Here's how the part is built. I have some questions about the finished solid (model axes, mm). Face numbers are marked on the shaded views. A direction names the side the tool comes from. Give positions to 0.01 mm unless a question says otherwise; leave off trailing zeros. Write each loop counter-clockwise with the first axis right and the second up, starting at its lowest first coordinate (ties: lowest second). Pieces come first, ordered by that corner, then holes. Notation, with made-up numbers: (-29, -26.75) -> (25, -26.75) arc R34 ccw to (25, 3.25) -> close; hole circle Ø11 at (-27.5, 88.25). An arc over 180 degrees is marked (long way). Use one line per item in the form item = value.
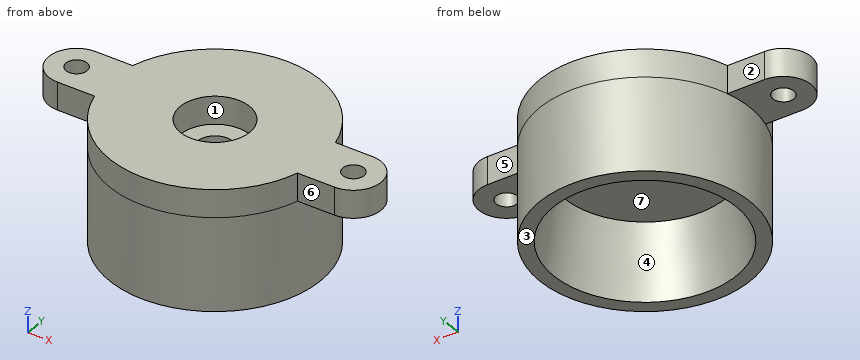
```python
from build123d import *

# Parameters (mm, degrees)
F0_R     = 24.13
F0_R_2   = 20.955
F1_DEPTH = 16.51
F2_R     = 18.415
F2_R_2   = 24.13
F4_DEPTH = 4.7625
F5_R     = 3.96875
F6_DEPTH = 4.7625
F5_R_2   = 2.413
F5_R_3   = 7.9375
F7_DEPTH = 6.35


# Not quite as in the source:
# - a feature names something its author has since deleted; it is built from what else it names


with BuildPart() as f1:
    # F0 (on Top) → F1 (new body)
    with BuildSketch(Plane.XY):
        Circle(F0_R)
        Circle(F0_R_2, mode=Mode.SUBTRACT)
        Circle(F0_R_2)
    extrude(amount=F1_DEPTH)

    # F0 (on Top) → F3 section 0
    with BuildSketch(Plane.XY):
        Circle(F0_R_2)
    # F2 (on face) → F3 section 1
    with BuildSketch(Plane.XY.offset(16.51)):
        Circle(F2_R)
    loft(mode=Mode.SUBTRACT)

    # F2 (on face) → F4 (join)
    with BuildSketch(Plane.XY.offset(16.51)):
        Circle(F2_R_2)
        Circle(F2_R, mode=Mode.SUBTRACT)
        Circle(F2_R)
    extrude(amount=F4_DEPTH)

    # F5 (on face) → F6 (cut, through all)
    with BuildSketch(Plane.XY.offset(21.2725)):
        Circle(F5_R)
    extrude(amount=-F6_DEPTH, mode=Mode.SUBTRACT)

    # F5 (on face) → F7 (join)
    with BuildSketch(Plane.XY.offset(21.2725)):
        with BuildLine():
            Line((-26.2298047315, 6.35), (-31.75, 6.35))
            ThreePointArc((-31.75, 6.35), (-38.1, 0), (-31.75, -6.35))
            Line((-31.75, -6.35), (-26.2298047315, -6.35))
            ThreePointArc((-26.2298047315, -6.35), (-26.9875, 0), (-26.2298047315, 6.35))
        make_face()
        with Locations((-31.75, 0)):
            Circle(F5_R_2, mode=Mode.SUBTRACT)
        with BuildLine():
            ThreePointArc((23.2794845304, 6.35), (0, 24.13), (-23.2794845304, 6.35))
            ThreePointArc((-23.2794845304, 6.35), (-24.13, 0), (-23.2794845304, -6.35))
            ThreePointArc((-23.2794845304, -6.35), (0, -24.13), (23.2794845304, -6.35))
            ThreePointArc((23.2794845304, -6.35), (23.9164259633, -3.2033527968), (24.13, 0))
            ThreePointArc((24.13, 0), (23.9164259633, 3.2033527968), (23.2794845304, 6.35))
        make_face()
        Circle(F5_R_3, mode=Mode.SUBTRACT)
        with BuildLine():
            Line((31.75, 6.35), (26.2298047315, 6.35))
            ThreePointArc((26.2298047315, 6.35), (26.9875, 0), (26.2298047315, -6.35))
            Line((26.2298047315, -6.35), (31.75, -6.35))
            ThreePointArc((31.75, -6.35), (38.1, 0), (31.75, 6.35))
        make_face()
        with Locations((31.75, 0)):
            Circle(F5_R_2, mode=Mode.SUBTRACT)
        with BuildLine():
            Line((-23.2794845304, 6.35), (-26.2298047315, 6.35))
            ThreePointArc((-26.2298047315, 6.35), (-26.9875, 0), (-26.2298047315, -6.35))
            Line((-26.2298047315, -6.35), (-23.2794845304, -6.35))
            ThreePointArc((-23.2794845304, -6.35), (-24.13, 0), (-23.2794845304, 6.35))
        make_face()
        with BuildLine():
            Line((26.2298047315, 6.35), (23.2794845304, 6.35))
            ThreePointArc((23.2794845304, 6.35), (23.9164259633, 3.2033527968), (24.13, 0))
            ThreePointArc((24.13, 0), (23.9164259633, -3.2033527968), (23.2794845304, -6.35))
            Line((23.2794845304, -6.35), (26.2298047315, -6.35))
            ThreePointArc((26.2298047315, -6.35), (26.9875, 0), (26.2298047315, 6.35))
        make_face()
    extrude(amount=F7_DEPTH)


solid = f1.part
```
Q1. I want a section at C-C, the plane z = 18. Write out the boundary of the cut face in (x, y), and give its area (3 significant figures).
Result set:
outline = circle Ø48.26 at (0, 0); hole circle Ø7.94 at (0, 0)
area = 1,780 mm2
Q2. I want a section at D-D, the plane z = 11. Write out the boundary of the cut face in (x, y), and give its area (3 significant figures).
Result set:
outline = circle Ø48.26 at (0, 0); hole circle Ø38.53 at (0, 0)
area = 664 mm2
Q3. Will these pins go through, and if not, where does the flat tip stop? pin 1 Ø8 at (x, z) = (-3, 20.5) entering from -Y; pin 2 Ø5.5 at (x, y) = (31.75, 0) entering from -Z; pin 3 Ø12 at (x, z) = (21, 22.5) entering from +Y.
Result set:
pin_1 = -24.13
pin_2 = 21.27
pin_3 = 18.9
Q4. I want a section at A-A, the plane x = 0. Write out the boundary of the cut face in (y, z) (1 decimal), and give its area (3 significant figures).
Result set:
outline = (-24.1, 0) -> (-21, 0) -> (-18.4, 16.5) -> (-4, 16.5) -> (-4, 21.3) -> (-7.9, 21.3) -> (-7.9, 27.6) -> (-24.1, 27.6) -> close; (4, 16.5) -> (18.4, 16.5) -> (21, 0) -> (24.1, 0) -> (24.1, 27.6) -> (7.9, 27.6) -> (7.9, 21.3) -> (4, 21.3) -> close
area = 544 mm2
Q5. If I drill on line 1 along Y through (x, z) = (0, 19.5); line 2 along Y through (x, z) = (0, 24.5); line 3 along X through (y, z) = (-2.5, 5.5), over which ranges is the centre line in solid material (lowest first)? Write a range as from..to.
Result set:
line_1 = -24.13..-3.97, 3.97..24.13
line_2 = -24.13..-7.94, 7.94..24.13
line_3 = -24..-19.95, 19.95..24
Q6. Which directions (+Z, -Z, +X, -X, +Y, -Y) give clear straight access to the entire face, cutting with the end or side of a thin tool? Please do the marked faces 5, 6 and 7.
Result set:
face_5 = +Z, -Z, +X, +Y
face_6 = +Z, -Z, +X, -Y
face_7 = -Z
Q7. I want a section at B-B, the plane y = 0. Count the separate pieces of the cut face and the enclosed holes in it, and give its area (3 significant figures).
Result set:
separate_pieces = 4
enclosed_holes = 0
area = 661 mm2
Q8. If we mould it in two halves opening along Y, with no side actions, what happens to the marked faces 1, 2, 3 and 4? For each: +Y half, -Y half, draft (parallel to the pull), parting line (faces both ways), or undercut.
Result set:
face_1 = undercut
face_2 = +Y half
face_3 = draft
face_4 = undercut
